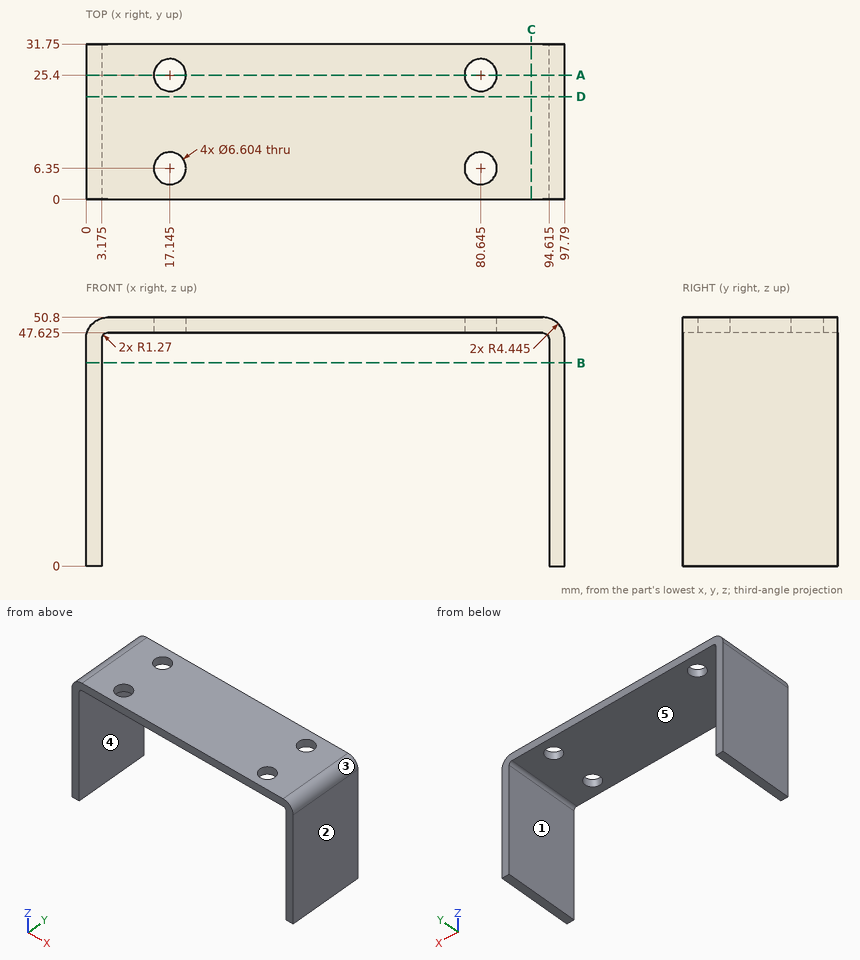
Input: dimensioned drawing with shaded views. Units: mm. Origin: part minimum x, y, z. A direction names the side the tool comes from. Coordinates: 2 decimals unless noted, no trailing zeros. Order: outer loops, then holes, each group sorted by start corner. A loop starts at its lowest first (then second) coordinate and runs counter-clockwise, first axis right, second up.
(1) First-contact query: pin 1 (4 mm diameter, centred on x = 17.145, y = 6.35, fed in from -Z); pin 2 (5 mm diameter, centred on x = 69, y = 21, fed in from -Z) (3 decimals); pin 3 (6 mm diameter, centred on y = 8.5, z = 39, fed in from -X). Flat tips, straight axial feed; report the tip coordinate or a pass-through.
(2) Section query B-B (z = 41.5). Return the cut outline in (x, y) (3 decimals).
(3) Section query D-D (y = 21). Return the cut outline in (x, z) (3 decimals), plus the area to 3 significant figures.
(4) Draft query along Z for the marked faces 3, 4 and 5. Return one class per face: pulls with the +Z half, pulls with the -Z half, needs draft (parallel to the pull), parting line crosses it, or undercut.
(5) Access query for the marked faces 1 and 2. Directions: +Z, -Z, +X, -X, +Y, -Y. A direction counts if a zero-diameter tool reaches every point of the face in a straight line with its end or side. Return the directions, or none.
(6) Section query A-A (y = 25.4). Return the cut outline in (x, z) (3 decimals), plus the area to 3 significant figures.
(7) Material intervals for probe 1 along X at (y, z) = (25, 37) (3 decimals); probe 2 along Z at (x, y) = (63, 11) (3 decimals); probe 3 along X at (y, z) = (6, 48), sorted ascending.
(8) Section query C-C (x = 91). Return the cut outline in (y, z) (3 decimals), plus the area to 3 significant figures.
Solution:
1. pin 1: passes through
1. pin 2: stops at z = 47.625
1. pin 3: stops at x = 0
2. outline: (0, 0) - (3.175, 0) - (3.175, 31.75) - (0, 31.75) - close; (94.615, 0) - (97.79, 0) - (97.79, 31.75) - (94.615, 31.75) - close
3. outline: (0, 0) - (3.175, 0) - (3.175, 46.355) arc R1.27 cw to (4.445, 47.625) - (93.345, 47.625) arc R1.27 cw to (94.615, 46.355) - (94.615, 0) - (97.79, 0) - (97.79, 46.355) arc R4.445 ccw to (93.345, 50.8) - (4.445, 50.8) arc R4.445 ccw to (0, 46.355) - close
3. area: 605 mm2
4. face 3: pulls with the +Z half
4. face 4: needs draft
4. face 5: pulls with the -Z half
5. face 1: -Z, +Y, -Y
5. face 2: +Z, -Z, +X, +Y, -Y
6. outline: (0, 0) - (3.175, 0) - (3.175, 46.355) arc R1.27 cw to (4.445, 47.625) - (13.843, 47.625) - (13.843, 50.8) - (4.445, 50.8) arc R4.445 ccw to (0, 46.355) - close; (20.447, 47.625) - (77.343, 47.625) - (77.343, 50.8) - (20.447, 50.8) - close; (83.947, 47.625) - (93.345, 47.625) arc R1.27 cw to (94.615, 46.355) - (94.615, 0) - (97.79, 0) - (97.79, 46.355) arc R4.445 ccw to (93.345, 50.8) - (83.947, 50.8) - close
6. area: 563 mm2
7. probe 1: x = 0 to 3.175, 94.615 to 97.79
7. probe 2: z = 47.625 to 50.8
7. probe 3: x = 0.32 to 13.86, 20.43 to 77.36, 83.93 to 97.47
8. outline: (0, 47.625) - (31.75, 47.625) - (31.75, 50.8) - (0, 50.8) - close
8. area: 101 mm2
